```python
from build123d import *

# Parameters (mm, degrees)
F0_R     = 40
F1_DEPTH = 20
F2_W     = 76.681012
F2_H     = 22.804
F3_DEPTH = 50
F4_W     = 76.681012
F4_H     = 12.157896
F5_DEPTH = 8
F6_R     = 4.262414
F7_DEPTH = 51.403


with BuildPart() as f1:
    # F0 (on Top) → F1 (new body)
    with BuildSketch(Plane.XY):
        Circle(F0_R)
    extrude(amount=F1_DEPTH)

    # F2 (on face) → F3 (join)
    with BuildSketch(Plane.XY.offset(20)):
        Rectangle(F2_W, F2_H)
    extrude(amount=F3_DEPTH)

    # F4 (on face) → F5 (cut)
    with BuildSketch(Plane.XY.offset(70)):
        Rectangle(F4_W, F4_H)
    extrude(amount=-F5_DEPTH, mode=Mode.SUBTRACT)

    # F6 (on face) → F7 (cut, through all)
    with BuildSketch(Plane(origin=(0, 11.402, 0), x_dir=(-1, 0, 0), z_dir=(0, 1, 0))):
        with Locations((-15.634964, 30)):
            Circle(F6_R)
        with Locations((15.634964, 30)):
            Circle(F6_R)
    extrude(amount=-F7_DEPTH, mode=Mode.SUBTRACT)


solid = f1.part
```
The listing builds one solid part. Answer for the finished solid, in the listing's coordinates (mm). A direction names the side the tool comes from. Coordinates: 2 decimals unless noted, no trailing zeros. Write each loop counter-clockwise with the first axis right and the second up, starting at its lowest first coordinate (ties: lowest second). Pieces come first, ordered by that corner, then holes. Notation, with made-up numbers: (28, 12.5) - (59, 12.5) arc R12 cw to (59, 16.5) - close; hole circle Ø4 at (42.25, 60.5). An arc over 180 degrees is marked (long way). Return JSON: item names as keys, results as strings. Group by question number.
1. A cutting plane is placed at C-C, the plane x = 15. Determine the outline of the cut face in (y, z).
2. A cutting plane is placed at B-B, the plane y = 0. Determine the outline of the cut face in (x, z), plus the area to 3 significant figures.
3. Given pin 1 (25 mm diameter, centred on x = -13.5, z = 45, fed in from +Y); pin 2 (7 mm diameter, centred on y = -1.5, z = 54.5, fed in from -X); pin 3 (4 mm diameter, centred on x = -22, z = 45, fed in from -Y); pin 4 (5 mm diameter, centred on x = -15.63, z = 30, fed in from -Y), each flat-ended and moving along its own axis, determine where each tip first touches the part or whether it passes through.
4. A cutting plane is placed at D-D, the plane x = 0. Determine the outline of the cut face in (y, z).
5. Straight lines are drawn through the part: L1, parallel to Y at x = -8, z = 64.5; L2, parallel to Z at x = -15.5, y = 29.5; L3, parallel to Y at x = 5.5, z = 20.5. For each, find the intervals that lie inside material, in ascending order.
6. Which of the six approach directions +Z, -Z, +X, -X, +Y, -Y give full straight-line access (tool end or side, diameter ignored) to faces 1 (the flat face through (-1, 0, 62)), 2 (the flat face through (38.341, 0, 45)), 3 (the flat face through (-1, -11.402, 45)), 4 (the flat face through (-1, 23, 20))?
7. Determine the mould class of faces 5 (the flat face through (-1, 6.079, 66)), 6 (the flat face through (-1, -22, 20)), 7 (the flat face through (-1, 1, 0)), 8 (the cylindrical face through (16.56, 0.16, 25.84)) for opening direction Z: released by +Z, released by -Z, zero draft, split by the parting line, or undercut.
8. A cutting plane is placed at A-A, the plane z = 30. Determine the outline of the cut face in (x, y).
Ans:
{
 "1": {"outline": "(-37.08, 0) - (37.08, 0) - (37.08, 20) - (11.4, 20) - (11.4, 25.79) - (-11.4, 25.79) - (-11.4, 20) - (-37.08, 20) - close; (-11.4, 34.21) - (11.4, 34.21) - (11.4, 70) - (6.08, 70) - (6.08, 62) - (-6.08, 62) - (-6.08, 70) - (-11.4, 70) - close"},
 "2": {"outline": "(-40, 0) - (40, 0) - (40, 20) - (38.34, 20) - (38.34, 62) - (-38.34, 62) - (-38.34, 20) - (-40, 20) - close; hole circle Ø8.52 at (-15.63, 30); hole circle Ø8.52 at (15.63, 30)", "area": "4,710 mm²"},
 "3": {"pin 1": "y = 11.4", "pin 2": "x = -38.34", "pin 3": "y = -11.4", "pin 4": "through"},
 "4": {"outline": "(-40, 0) - (40, 0) - (40, 20) - (11.4, 20) - (11.4, 70) - (6.08, 70) - (6.08, 62) - (-6.08, 62) - (-6.08, 70) - (-11.4, 70) - (-11.4, 20) - (-40, 20) - close"},
 "5": {"L1": "-11.4 to -6.08, 6.08 to 11.4", "L2": "0 to 20", "L3": "-11.4 to 11.4"},
 "6": {"face 1": "+Z, +X, -X", "face 2": "+Z, +X, +Y, -Y", "face 3": "+Z, +X, -X, -Y", "face 4": "+Z, +X, -X, +Y"},
 "7": {"face 5": "zero draft", "face 6": "released by +Z", "face 7": "released by -Z", "face 8": "undercut"},
 "8": {"outline": "(-38.34, -11.4) - (-19.9, -11.4) - (-19.9, 11.4) - (-38.34, 11.4) - close; (-11.37, -11.4) - (11.37, -11.4) - (11.37, 11.4) - (-11.37, 11.4) - close; (19.9, -11.4) - (38.34, -11.4) - (38.34, 11.4) - (19.9, 11.4) - close"}
}
